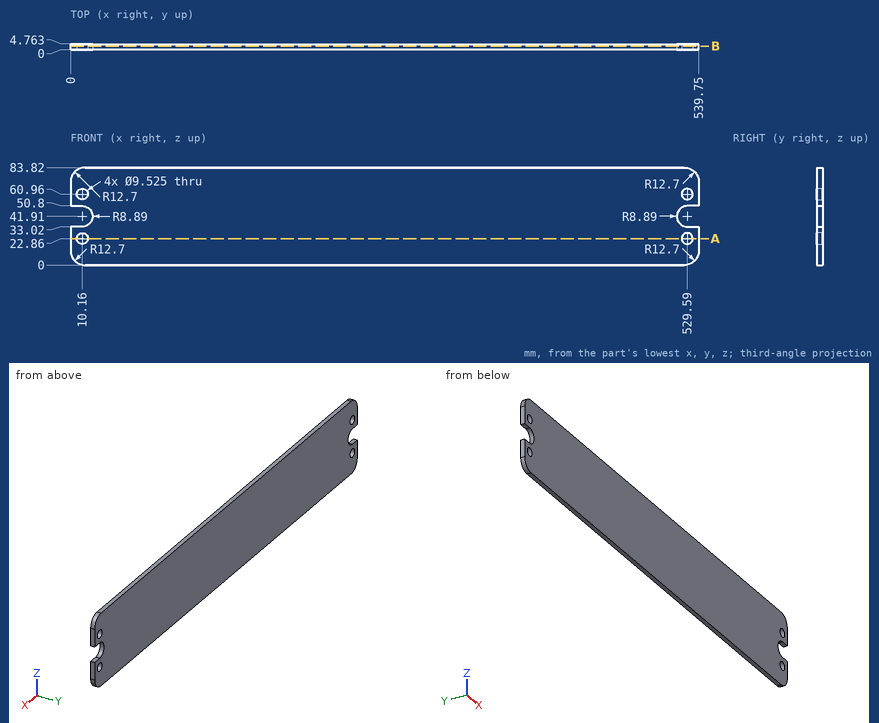
Geometry: see drawing. Coordinates: mm, zero at the bounding-box minimum. Round coordinates to 2 decimals unless told otherwise and drop trailing zeros. Loops run counter-clockwise (first coordinate to the right, second up) from the corner with the lowest first, then second, coordinate; pieces in that order, holes last. Notation, with made-up numbers: (-19.75, -34) - (21.25, -34) arc R38 cw to (21.25, 5) - close; hole circle Ø6 at (44, -38.5). An arc over 180 degrees is marked (long way). Write item = value, one per line. Start each with the question number.
(1) Ray query, line 1 along X through (y, z) = (2.1, 22.86); line 2 along Z through (x, y) = (529.59, 3.85); line 3 along X through (y, z) = (1.9, 63.5). Return the intervals inside material, ascending. Write a range as from..to.
(2) Pin query (flat end, axial travel): pin 1 (7.5 mm diameter, centred on x = 10.16, z = 22.86, fed in from +Y); pin 2 (1.4 mm diameter, centred on x = 5, y = 2, fed in from +Z); pin 3 (1.4 mm diameter, centred on x = 532, y = 1.5, fed in from -Z); pin 4 (2.5 mm diameter, centred on x = 5.5, y = 2.5, fed in from -Z). Return the tip coordinate at first contact, or that it passes through.
(3) Section query A-A, the plane z = 22.86. Output: boundary loops of the cut face in (x, y), plus the area to 3 significant figures.
(4) Section query B-B, the plane y = 2.95. State how many separate pieces and enclosed holes the cut face has, plus the area to 3 significant figures.
Conclusion:
q1.line_1 = 0..5.4, 14.92..524.83, 534.35..539.75
q1.line_2 = 0.26..18.1, 27.62..33.02, 50.8..56.2, 65.72..83.56
q1.line_3 = 0..6.13, 14.19..525.56, 533.62..539.75
q2.pin_1 = through
q2.pin_2 = 81.72
q2.pin_3 = 0.73
q2.pin_4 = 1.48
q3.outline = (0, 0) - (5.4, 0) - (5.4, 4.76) - (0, 4.76) - close; (14.92, 0) - (524.83, 0) - (524.83, 4.76) - (14.92, 4.76) - close; (534.35, 0) - (539.75, 0) - (539.75, 4.76) - (534.35, 4.76) - close
q3.area = 2,480 mm2
q4.separate_pieces = 1
q4.enclosed_holes = 4
q4.area = 44,200 mm2
